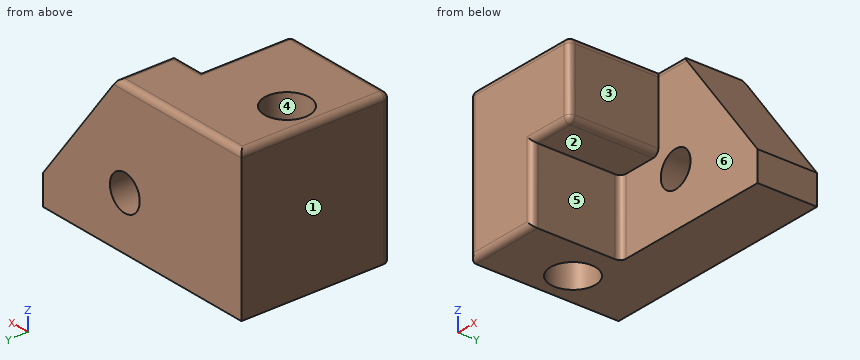
from build123d import *

# Parameters (mm, degrees)
F0_W     = 203.2
F0_H     = 127
F1_DEPTH = 127
F3_DEPTH = 76.2
F4_SIZE2 = 101.6
F4_SIZE  = 76.2
F5_R     = 5.08
F6_R     = 15.24
F7_DEPTH = 50.8
F8_R     = 19.05
F9_DEPTH = 127


with BuildPart() as f1:
    # F0 (on Front) → F1 (new body)
    with BuildSketch(Plane.XZ):
        with Locations((-8.7118318382, 17.0372370631)):
            Rectangle(F0_W, F0_H)
    extrude(amount=F1_DEPTH)

    # F2 (on face) → F3 (cut)
    with BuildSketch(Plane.XZ.offset(127)):
        Polygon((92.8881681618, 80.5372370631), (-8.7118318382, 80.5372370631), (-8.7118318382, 17.0372370631), (-46.8118318382, 17.0372370631), (-46.8118318382, -46.4627629369), (92.8881681618, -46.4627629369), align=None)
    extrude(amount=-F3_DEPTH, mode=Mode.SUBTRACT)

    # F4
    f4_edges = [f1.edges().sort_by_distance(p)[0] for p in [
        (92.888168, -25.4, 80.537237),
    ]]
    f4_side = f1.faces().sort_by_distance((-30.48326, -52.614286, 80.537237))[0]
    chamfer(f4_edges, length=F4_SIZE, length2=F4_SIZE2, reference=f4_side)

    # F5
    f5_edges = [f1.edges().sort_by_distance(p)[0] for p in [
        (-8.711832, -88.9, 80.537237),
        (3.988168, -50.8, 80.537237),
        (-8.711832, -88.9, 17.037237),
        (-8.711832, -127, 48.787237),
        (-27.761832, -127, 17.037237),
        (-46.811832, -127, -14.712763),
        (-78.561832, -127, -46.462763),
        (-110.311832, -127, 17.037237),
        (-59.511832, -127, 80.537237),
        (-46.811832, -50.8, -14.712763),
        (16.688168, -25.4, 80.537237),
        (-46.811832, 0, 80.537237),
        (-110.311832, -63.5, 80.537237),
    ]]
    fillet(f5_edges, radius=F5_R)

    # F6 (on face) → F7 (cut, through all)
    with BuildSketch(Plane.XZ.offset(50.8)):
        with Locations((9.0681681618, -0.7427629369)):
            Circle(F6_R)
    extrude(amount=-F7_DEPTH, mode=Mode.SUBTRACT)

    # F8 (on face) → F9 (cut, through all)
    with BuildSketch(Plane.XY.offset(80.5372370631)):
        with Locations((-82.0436404108, -62.4904338136)):
            Circle(F8_R)
    extrude(amount=-F9_DEPTH, mode=Mode.SUBTRACT)


solid = f1.part
The listing builds one solid part. Answer for the finished solid, in the listing's coordinates (mm). Face numbers are marked on the shaded views. A direction names the side the tool comes from. Give positions to 0.01 mm unless a question says otherwise; leave off trailing zeros. Loops run counter-clockwise (first coordinate to the right, second up) from the corner with the lowest first, then second, coordinate; pieces in that order, holes last.
Item 1: A cutting plane is placed at B-B (x = -96). Give the vertices of the cut face in (y, z), then the cut area to 3 significant figures.
Derived:
outline: (-127, -41.38) arc R5.08 ccw to (-121.92, -46.46) - (-75.46, -46.46) - (-75.46, 80.54) - (-121.92, 80.54) arc R5.08 ccw to (-127, 75.46) - close; (-49.52, -46.46) - (0, -46.46) - (0, 75.46) arc R5.08 ccw to (-5.08, 80.54) - (-49.52, 80.54) - close
area: 12,800 mm2
Item 2: Each of these flat-tipped pins is pushed along its axis until it touches: pin 1 Ø4 at (x, z) = (36.5, -30.5) entering from -Y; pin 2 Ø12 at (x, y) = (-87, -69) entering from -Z. Where does it stop, or does it pass through?
Derived:
pin 1: stops at y = -50.8
pin 2: passes through
Item 3: A cutting plane is placed at D-D (y = -11). Give the vertices of the cut face in (x, z), then the cut area to 3 significant figures.
Derived:
outline: (-110.31, -46.46) - (92.89, -46.46) - (92.89, -21.06) - (18.21, 78.51) arc R5.08 ccw to (14.15, 80.54) - (-105.23, 80.54) arc R5.08 ccw to (-110.31, 75.46) - close; hole circle Ø30.48 at (9.07, -0.74)
area: 21,200 mm2
Item 4: Find the intervals of material crossed by line 1 along Z through (x, y) = (10, -24); line 2 along X through (y, z) = (-118.5, 46.5); line 3 along Z through (x, y) = (-40, -72), in increasing order.
Derived:
line 1: z = -46.46 to -15.95, 14.47 to 80.54
line 2: x = -110.31 to -8.71
line 3: z = 17.04 to 80.54
Item 5: A cutting plane is placed at A-A (z = -3). Give the vertices of the cut face in (x, y).
Derived:
outline: (-110.31, -121.92) arc R5.08 ccw to (-105.23, -127) - (-51.89, -127) arc R5.08 ccw to (-46.81, -121.92) - (-46.81, -55.88) arc R5.08 cw to (-41.73, -50.8) - (-6, -50.8) - (-6, 0) - (-110.31, 0) - close; (24.14, -50.8) - (79.34, -50.8) - (79.34, 0) - (24.14, 0) - close; hole circle Ø38.1 at (-82.04, -62.49)
Item 6: Determine the mould class of the marked faces 4, 5 and 6 for opening direction Y: +Y half, -Y half, draft (parallel to the pull), parting line (faces both ways), or undercut.
Derived:
face 4: undercut
face 5: draft
face 6: -Y half
Item 7: A tool of negligible diameter and unlimited length cuts with its end or side. For the marked faces 1, 2 and 3, from which of +Z, -Z, +X, -X, +Y, -Y can it reach the whole face along a straight path? Write none if from no direction.
Derived:
face 1: +Z, -Z, -X, +Y, -Y
face 2: -Z, +X, -Y
face 3: +Z, -Z, +X, -Y
Item 8: A cutting plane is placed at C-C (x = -35). Give the vertices of the cut face in (y, z), then the cut area to 3 significant figures.
Derived:
outline: (-127, 22.12) arc R5.08 ccw to (-121.92, 17.04) - (-50.8, 17.04) - (-50.8, -46.46) - (0, -46.46) - (0, 75.46) arc R5.08 ccw to (-5.08, 80.54) - (-121.92, 80.54) arc R5.08 ccw to (-127, 75.46) - close
area: 11,300 mm2
